```python
from build123d import *

# Parameters (mm, degrees)
BOSS_EXTRUDE1_DEPTH = 127
SKETCH2_R           = 2.0828
CUT_EXTRUDE1_DEPTH  = 150.326295407
SKETCH3_R           = 2.0828
CUT_EXTRUDE2_DEPTH  = 5.08


with BuildPart() as part:
    # Sketch1 → Boss-Extrude1 (new, symmetric)
    with BuildSketch(Plane(origin=(0, 0, 0), x_dir=(0, 0, -1), z_dir=(1, 0, 0))):
        Polygon((-13.97, 33.02), (19.05, 33.02), (19.05, 38.1), (-19.05, 38.1), (-19.05, -38.1), (19.05, -38.1), (19.05, -33.02), (-13.97, -33.02), align=None)
    extrude(amount=BOSS_EXTRUDE1_DEPTH, both=True)

    # Sketch2 → Cut-Extrude1 (cut, through all)
    with BuildSketch(Plane(origin=(0, 38.1, 0), x_dir=(1, 0, 0), z_dir=(0, 1, 0))):
        with Locations(Location((-114.3, -0.945134, 0), (0, 0, 270))):
            Circle(SKETCH2_R)
        with Locations(Location((-101.6, -0.945134, 0), (0, 0, 270))):
            Circle(SKETCH2_R)
        with Locations(Location((-88.9, -0.945134, 0), (0, 0, 270))):
            Circle(SKETCH2_R)
        with Locations(Location((-76.2, -0.945134, 0), (0, 0, 270))):
            Circle(SKETCH2_R)
        with Locations(Location((-63.5, -0.945134, 0), (0, 0, 270))):
            Circle(SKETCH2_R)
        with Locations(Location((-50.8, -0.945134, 0), (0, 0, 270))):
            Circle(SKETCH2_R)
        with Locations(Location((-38.1, -0.945134, 0), (0, 0, 270))):
            Circle(SKETCH2_R)
        with Locations(Location((-25.4, -0.945134, 0), (0, 0, 270))):
            Circle(SKETCH2_R)
        with Locations(Location((-12.7, -0.945134, 0), (0, 0, 270))):
            Circle(SKETCH2_R)
        with Locations(Location((0, -0.945134, 0), (0, 0, 270))):
            Circle(SKETCH2_R)
        with Locations(Location((12.7, -0.945134, 0), (0, 0, 270))):
            Circle(SKETCH2_R)
        with Locations(Location((25.4, -0.945134, 0), (0, 0, 270))):
            Circle(SKETCH2_R)
        with Locations(Location((38.1, -0.945134, 0), (0, 0, 270))):
            Circle(SKETCH2_R)
        with Locations(Location((50.8, -0.945134, 0), (0, 0, 270))):
            Circle(SKETCH2_R)
        with Locations(Location((63.5, -0.945134, 0), (0, 0, 270))):
            Circle(SKETCH2_R)
        with Locations(Location((76.2, -0.945134, 0), (0, 0, 270))):
            Circle(SKETCH2_R)
        with Locations(Location((88.9, -0.945134, 0), (0, 0, 270))):
            Circle(SKETCH2_R)
        with Locations(Location((101.6, -0.945134, 0), (0, 0, 270))):
            Circle(SKETCH2_R)
        with Locations(Location((114.3, -0.945134, 0), (0, 0, 270))):
            Circle(SKETCH2_R)
    extrude(amount=-CUT_EXTRUDE1_DEPTH, mode=Mode.SUBTRACT)

    # Sketch3 → Cut-Extrude2 (cut)
    with BuildSketch(Plane.XY.offset(19.05)):
        with Locations((-114.3, 17.78)):
            Circle(SKETCH3_R)
        with Locations((-101.6, 17.78)):
            Circle(SKETCH3_R)
        with Locations((-88.9, 17.78)):
            Circle(SKETCH3_R)
        with Locations((-76.2, 17.78)):
            Circle(SKETCH3_R)
        with Locations((-63.5, 17.78)):
            Circle(SKETCH3_R)
        with Locations((-50.8, 17.78)):
            Circle(SKETCH3_R)
        with Locations((-38.1, 17.78)):
            Circle(SKETCH3_R)
        with Locations((-25.4, 17.78)):
            Circle(SKETCH3_R)
        with Locations((-12.7, 17.78)):
            Circle(SKETCH3_R)
        with Locations((0, 17.78)):
            Circle(SKETCH3_R)
        with Locations((12.7, 17.78)):
            Circle(SKETCH3_R)
        with Locations((25.4, 17.78)):
            Circle(SKETCH3_R)
        with Locations((38.1, 17.78)):
            Circle(SKETCH3_R)
        with Locations((50.8, 17.78)):
            Circle(SKETCH3_R)
        with Locations((63.5, 17.78)):
            Circle(SKETCH3_R)
        with Locations((76.2, 17.78)):
            Circle(SKETCH3_R)
        with Locations((88.9, 17.78)):
            Circle(SKETCH3_R)
        with Locations((101.6, 17.78)):
            Circle(SKETCH3_R)
        with Locations((114.3, 17.78)):
            Circle(SKETCH3_R)
        with Locations((-101.6, 5.08)):
            Circle(SKETCH3_R)
        with Locations((-88.9, 5.08)):
            Circle(SKETCH3_R)
        with Locations((-76.2, 5.08)):
            Circle(SKETCH3_R)
        with Locations((-63.5, 5.08)):
            Circle(SKETCH3_R)
        with Locations((-50.8, 5.08)):
            Circle(SKETCH3_R)
        with Locations((-38.1, 5.08)):
            Circle(SKETCH3_R)
        with Locations((-25.4, 5.08)):
            Circle(SKETCH3_R)
        with Locations((-12.7, 5.08)):
            Circle(SKETCH3_R)
        with Locations((0, 5.08)):
            Circle(SKETCH3_R)
        with Locations((12.7, 5.08)):
            Circle(SKETCH3_R)
        with Locations((25.4, 5.08)):
            Circle(SKETCH3_R)
        with Locations((38.1, 5.08)):
            Circle(SKETCH3_R)
        with Locations((50.8, 5.08)):
            Circle(SKETCH3_R)
        with Locations((63.5, 5.08)):
            Circle(SKETCH3_R)
        with Locations((76.2, 5.08)):
            Circle(SKETCH3_R)
        with Locations((88.9, 5.08)):
            Circle(SKETCH3_R)
        with Locations((101.6, 5.08)):
            Circle(SKETCH3_R)
        with Locations((114.3, 5.08)):
            Circle(SKETCH3_R)
        with Locations((-101.6, -7.62)):
            Circle(SKETCH3_R)
        with Locations((-88.9, -7.62)):
            Circle(SKETCH3_R)
        with Locations((-76.2, -7.62)):
            Circle(SKETCH3_R)
        with Locations((-63.5, -7.62)):
            Circle(SKETCH3_R)
        with Locations((-50.8, -7.62)):
            Circle(SKETCH3_R)
        with Locations((-38.1, -7.62)):
            Circle(SKETCH3_R)
        with Locations((-25.4, -7.62)):
            Circle(SKETCH3_R)
        with Locations((-12.7, -7.62)):
            Circle(SKETCH3_R)
        with Locations((0, -7.62)):
            Circle(SKETCH3_R)
        with Locations((12.7, -7.62)):
            Circle(SKETCH3_R)
        with Locations((25.4, -7.62)):
            Circle(SKETCH3_R)
        with Locations((38.1, -7.62)):
            Circle(SKETCH3_R)
        with Locations((50.8, -7.62)):
            Circle(SKETCH3_R)
        with Locations((63.5, -7.62)):
            Circle(SKETCH3_R)
        with Locations((76.2, -7.62)):
            Circle(SKETCH3_R)
        with Locations((88.9, -7.62)):
            Circle(SKETCH3_R)
        with Locations((101.6, -7.62)):
            Circle(SKETCH3_R)
        with Locations((114.3, -7.62)):
            Circle(SKETCH3_R)
        with Locations((-114.3, 5.08)):
            Circle(SKETCH3_R)
        with Locations((-114.3, -7.62)):
            Circle(SKETCH3_R)
    extrude(amount=-CUT_EXTRUDE2_DEPTH, mode=Mode.SUBTRACT)


solid = part.part
```
Work out the finished part from the listing and answer in its coordinate system (mm). Round coordinates to 2 decimals unless told otherwise and drop trailing zeros. Loops run counter-clockwise (first coordinate to the right, second up) from the corner with the lowest first, then second, coordinate; pieces in that order, holes last. Notation, with made-up numbers: M 38,79 L 88,79 A33 ccw 88,118 Z; hole C 4,25.25 d5. An arc over 180 degrees is marked long. Use CSV: the item, a comma, the result in double quotes.
Q1. Section C-C, the plane y = 28 is taken. Determine the outline of the cut face in (x, z), then the cut area to 3 significant figures.
Determined:
outline,"M -127,13.97 L 127,13.97 L 127,19.05 L -127,19.05 Z"
area,"1,290 mm2"
Q2. Section A-A, the plane z = -13 is taken. Determine the outline of the cut face in (x, y), then the cut area to 3 significant figures.
Determined:
outline,"M -127,-38.1 L 127,-38.1 L 127,-33.02 L -127,-33.02 Z; M -127,33.02 L 127,33.02 L 127,38.1 L -127,38.1 Z"
area,"2,580 mm2"
Q3. Each of these flat-tipped pins is pushed along its axis until it touches: pin 1 (5 mm diameter, centred on x = 50.8, z = 0.95, fed in from -Y); pin 2 (5 mm diameter, centred on x = -101.6, y = -7.62, fed in from -Z); pin 3 (3.5 mm diameter, centred on x = 50.8, y = -7.62, fed in from -Z). Where does it stop, or does it pass through?
Determined:
pin 1,"y = -38.1"
pin 2,"z = 13.97"
pin 3,"through"
Q4. Consider L1, parallel to Y at x = 114.3, z = 15.1; L2, parallel to Y at x = 78, z = 3; L3, parallel to Z at x = 112.5, y = 25. Determine where each line is inside the solid, lowest interval first.
Determined:
L1,"-38.1 to -9.7, -5.54 to 3, 7.16 to 15.7, 19.86 to 38.1"
L2,"-38.1 to -33.02, 33.02 to 38.1"
L3,"13.97 to 19.05"
Q5. Section B-B, the plane x = 31 is taken. Determine the outline of the cut face in (y, z), then the cut area to 3 significant figures.
Determined:
outline,"M -38.1,-19.05 L -33.02,-19.05 L -33.02,13.97 L 33.02,13.97 L 33.02,-19.05 L 38.1,-19.05 L 38.1,19.05 L -38.1,19.05 Z"
area,"723 mm2"
